Check sheet for the modelled part. Datum: model origin and axes. Units: mm. Face numbers are marked on the shaded views. A direction names the side the tool comes from. Round coordinates to 2 decimals unless told otherwise and drop trailing zeros. Order: outer loops, then holes, each group sorted by start corner. A loop starts at its lowest first (then second) coordinate and runs counter-clockwise, first axis right, second up. Notation, with made-up numbers: (18, 4.5) -> (38, 4.5) arc R14 cw to (38, 26.5) -> close; hole circle Ø10 at (-17, 24). An arc over 180 degrees is marked (long way). Answer in a Markdown table with one row per item.
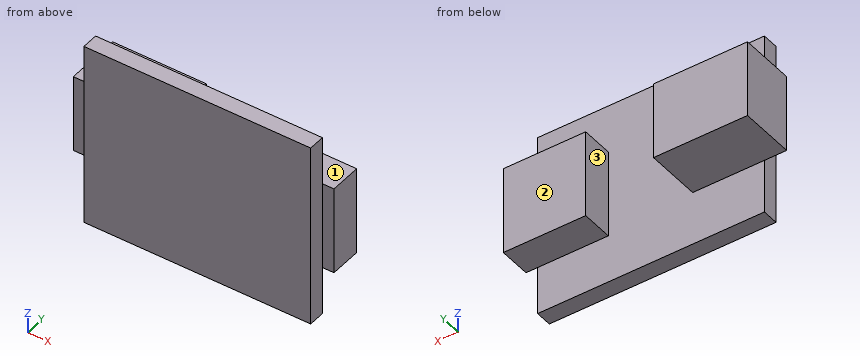
```python
from build123d import *

# Parameters (mm, degrees)
SKETCH1_W           = 23.4
SKETCH1_H           = 19.1
BOSS_EXTRUDE1_DEPTH = 1.7
SKETCH2_W           = 7.3
SKETCH2_H           = 9.1
BOSS_EXTRUDE2_DEPTH = 3.3
SKETCH3_W           = 9.1
SKETCH3_H           = 3.3
BOSS_EXTRUDE3_DEPTH = 1.2
SKETCH4_W           = 7.4
SKETCH4_H           = 8
BOSS_EXTRUDE5_DEPTH = 5.7
SKETCH5_W           = 8
SKETCH5_H           = 5.7
BOSS_EXTRUDE6_DEPTH = 2.3


with BuildPart() as part:
    # Sketch1 → Boss-Extrude1 (new body)
    with BuildSketch(Plane(origin=(0, 0, 0), x_dir=(1, 0, 0), z_dir=(0, 1, 0))):
        Rectangle(SKETCH1_W, SKETCH1_H)
    extrude(amount=BOSS_EXTRUDE1_DEPTH)

    # Sketch2 → Boss-Extrude2 (add)
    with BuildSketch(Plane(origin=(0, 1.7, 0), x_dir=(1, 0, 0), z_dir=(0, 1, 0))):
        with Locations((8.05, 0)):
            Rectangle(SKETCH2_W, SKETCH2_H)
    extrude(amount=BOSS_EXTRUDE2_DEPTH)

    # Sketch3 → Boss-Extrude3 (add)
    with BuildSketch(Plane(origin=(11.7, 0, 0), x_dir=(0, 0, -1), z_dir=(1, 0, 0))):
        with Locations((0, 3.35)):
            Rectangle(SKETCH3_W, SKETCH3_H)
    extrude(amount=BOSS_EXTRUDE3_DEPTH)

    # Sketch4 → Boss-Extrude5 (add)
    with BuildSketch(Plane(origin=(0, 1.7, 0), x_dir=(1, 0, 0), z_dir=(0, 1, 0))):
        with Locations((-8, -0.05)):
            Rectangle(SKETCH4_W, SKETCH4_H)
    extrude(amount=BOSS_EXTRUDE5_DEPTH)

    # Sketch5 → Boss-Extrude6 (add)
    with BuildSketch(Plane.ZY.offset(11.7)):
        with Locations((0.05, 4.55)):
            Rectangle(SKETCH5_W, SKETCH5_H)
    extrude(amount=BOSS_EXTRUDE6_DEPTH)


solid = part.part
```
(1) Section check A-A on x = 9.75. Record the boundary of the cut face in (y, z), plus the area to 3 significant figures.
Solutions:
| item | result |
|---|---|
| outline | (0, -9.55) -> (1.7, -9.55) -> (1.7, -4.55) -> (5, -4.55) -> (5, 4.55) -> (1.7, 4.55) -> (1.7, 9.55) -> (0, 9.55) -> close |
| area | 62.5 mm^2 |
(2) Scan lines: probe 1 along X at (y, z) = (3.75, -2.5); probe 2 along Y at (x, z) = (-6.75, 7.5); probe 3 along X at (y, z) = (6.75, 2.75). Record each from-to range of solid material in increasing order. Write a range as from..to.
Solutions:
| item | result |
|---|---|
| probe 1 | -14..-4.3, 4.4..12.9 |
| probe 2 | 0..1.7 |
| probe 3 | -14..-4.3 |
(3) Section check B-B on z = 0.25. Record the boundary of the cut face in (x, y), plus the area to 3 significant figures.
Solutions:
| item | result |
|---|---|
| outline | (-14, 1.7) -> (-11.7, 1.7) -> (-11.7, 0) -> (11.7, 0) -> (11.7, 1.7) -> (12.9, 1.7) -> (12.9, 5) -> (4.4, 5) -> (4.4, 1.7) -> (-4.3, 1.7) -> (-4.3, 7.4) -> (-14, 7.4) -> close |
| area | 123 mm^2 |
(4) Depth check by flat-ended pin: pin 1 Ø3 at (x, z) = (3, -1.5) entering from +Y; pin 2 Ø1 at (x, y) = (7.5, 2.5) entering from +Z; pin 3 Ø1 at (x, y) = (8, 4) entering from -Z. Enter the tip coordinate at first touch or a pass-through.
Solutions:
| item | result |
|---|---|
| pin 1 | y = 5 |
| pin 2 | z = 4.55 |
| pin 3 | z = -4.55 |
(5) Section check C-C on y = 1.25. Record the boundary of the cut face in (x, z), plus the area to 3 significant figures.
Solutions:
| item | result |
|---|---|
| outline | (-11.7, -9.55) -> (11.7, -9.55) -> (11.7, 9.55) -> (-11.7, 9.55) -> close |
| area | 447 mm^2 |
(6) Tool access check on the marked faces 1, 2 and 3. Record the directions out of +Z, -Z, +X, -X, +Y, -Y that give a thin tool (end or side, any length) a straight path to the whole face; none if there is none.
Solutions:
| item | result |
|---|---|
| face 1 | +Z, +X, -X, +Y |
| face 2 | +Z, -Z, +X, +Y |
| face 3 | +Z, -Z, +Y |
(7) Section check D-D on x = -4.75. Record the boundary of the cut face in (y, z), plus the area to 3 significant figures.
Solutions:
| item | result |
|---|---|
| outline | (0, -9.55) -> (1.7, -9.55) -> (1.7, -3.95) -> (7.4, -3.95) -> (7.4, 4.05) -> (1.7, 4.05) -> (1.7, 9.55) -> (0, 9.55) -> close |
| area | 78.1 mm^2 |
